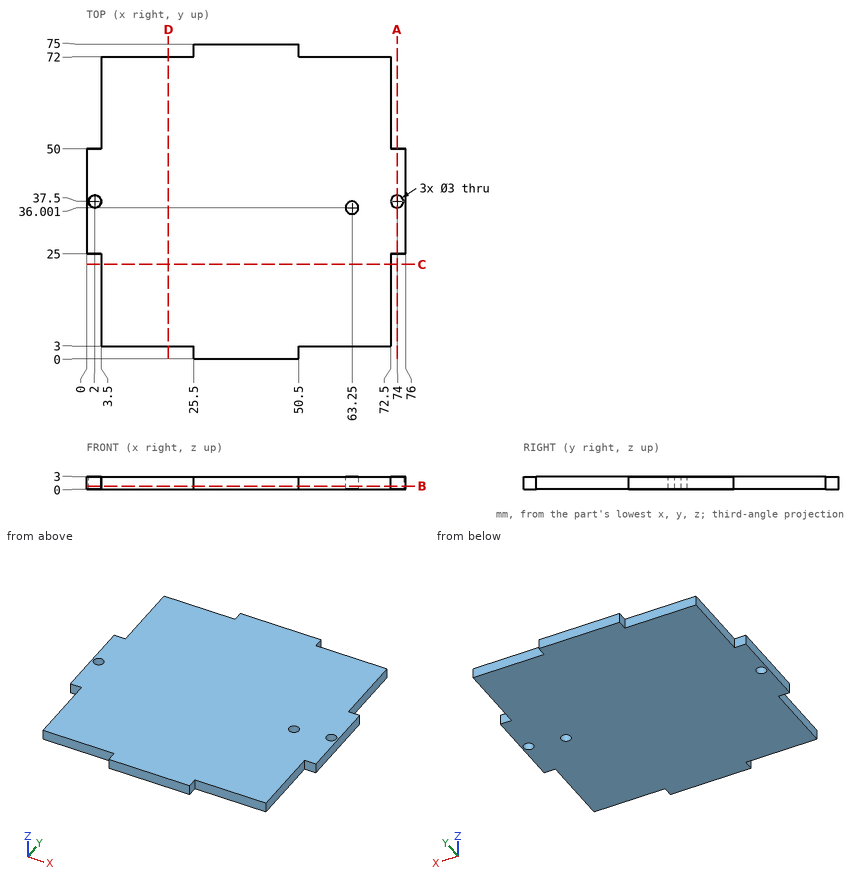
Job drawing, mm, ordinate dimensions from the low corner. One solid piece. Give positions to 0.01 mm unless a question says otherwise; leave off trailing zeros. Write each loop counter-clockwise with the first axis right and the second up, starting at its lowest first coordinate (ties: lowest second). Pieces come first, ordered by that corner, then holes. Notation, with made-up numbers: (71.25, 8.5) - (86.25, 8.5) arc R13 cw to (86.25, 12.5) - close; hole circle Ø4 at (12.25, 66). An arc over 180 degrees is marked (long way). Answer as CSV lines item,"result".
1. Drill centre lines: L1, parallel to Y at x = 74, z = 0.75; L2, parallel to X at y = 36.5, z = 0.5 (1 decimal); L3, parallel to Y at x = 24, z = 1.25. Where is each one in solid material? Low to high. Write a range as [from, to].
Responses:
L1,"y = [25, 36], [39, 50]"
L2,"x = [0, 0.9], [3.1, 61.8], [64.7, 72.9], [75.1, 76]"
L3,"y = [3, 72]"
2. Band-saw the part on C-C (y = 22.5). Write the cut outline in (x, z), and give its area (3 significant figures).
Responses:
outline,"(3.5, 0) - (72.5, 0) - (72.5, 3) - (3.5, 3) - close"
area,"207 mm2"
3. Band-saw the part on D-D (x = 19.5). Write the cut outline in (y, z), and give its area (3 significant figures).
Responses:
outline,"(3, 0) - (72, 0) - (72, 3) - (3, 3) - close"
area,"207 mm2"
4. Pin check, flat tips, straight feed: pin 1 (2.5 mm diameter, centred on x = 2, y = 37.5, fed in from -Z); pin 2 (0.9 mm diameter, centred on y = 73.5, z = 2, fed in from -X); pin 3 (1.5 mm diameter, centred on y = 63, z = 2, fed in from +X); pin 4 (1.5 mm diameter, centred on x = 56.5, z = 1.5, fed in from -Y). Stop position of each tip, or through.
Responses:
pin 1,"passes through"
pin 2,"stops at x = 25.5"
pin 3,"stops at x = 72.5"
pin 4,"stops at y = 3"
5. Band-saw the part on A-A (x = 74). Write the cut outline in (y, z), and give its area (3 significant figures).
Responses:
outline,"(25, 0) - (36, 0) - (36, 3) - (25, 3) - close; (39, 0) - (50, 0) - (50, 3) - (39, 3) - close"
area,"66.0 mm2"
6. Band-saw the part on B-B (z = 0.8). Write the cut outline in (x, y), and give its area (4 significant figures).
Responses:
outline,"(0, 25) - (3.5, 25) - (3.5, 3) - (25.5, 3) - (25.5, 0) - (50.5, 0) - (50.5, 3) - (72.5, 3) - (72.5, 25) - (76, 25) - (76, 50) - (72.5, 50) - (72.5, 72) - (50.5, 72) - (50.5, 75) - (25.5, 75) - (25.5, 72) - (3.5, 72) - (3.5, 50) - (0, 50) - close; hole circle Ø3 at (2, 37.5); hole circle Ø3 at (63.25, 36); hole circle Ø3 at (74, 37.5)"
area,"5,065 mm2"
